Autodesk Inventor part; units mm, degrees
ref_plane "YZ Plane" through (0, 0, 0) normal (1, 0, 0) x (0, 1, 0)
ref_plane "XZ Plane" through (0, 0, 0) normal (0, 1, 0) x (-1, 0, 0)
ref_plane "XY Plane" through (0, 0, 0) normal (0, 0, 1) x (1, 0, 0)
sketch "Sketch1" plane through (0, 0, 0) normal (0, 0, 1) x (1, 0, 0)
  circle A0 centre (0, 0) radius 3.5
  dimension "d0" = 7
extrude "Extrusion1" add sketch "Sketch1" along normal blind 15
fillet "Fillet1" radius 2 1 edges at (-3.5, 0, 15)
hole "Hole1" at (0, 0, 0) direction (0, 0, 1) diameter 3.25 end through all
properties part number "Landing Gear"
Model file for the job. Use its own axes, mm. Give positions to 0.01 mm unless a question says otherwise; leave off trailing zeros. Order: outer loops, then holes, each group sorted by start corner. A loop starts at its lowest first (then second) coordinate and runs counter-clockwise, first axis right, second up. Notation, with made-up numbers: M -5.5,3.5 L 46.5,3.5 A23 ccw 46.5,23.5 Z; hole C -30,-39 d11. An arc over 180 degrees is marked long. Put each result on its own line as item: value. Start each with the question number.
(1) Pin check, flat tips, straight feed: pin 1 Ø1.5 at (x, z) = (1, 6) entering from +Y; pin 2 Ø1 at (x, z) = (-1.5, 8) entering from +Y; pin 3 Ø1 at (x, z) = (-2, 13) entering from +Y. Stop position of each tip, or through.
(2) Pull direction X, two halves, no side cores. Call faces 1 (the face through (0.99, -1.29, 7.6)), 2 (the face through (1, -2, 0)), 3 (the face through (3.233, 1.341, 6.409)): released by +X, released by -X, zero draft, split by the parting line, or undercut.
(3) Band-saw the part on A-A on z = 4. Give the cut face in (x, y) (3 decimals), then the cut area to 3 significant figures.
(4) Drill centre lines: L1, parallel to Y at x = 0, z = 8.75 (3 decimals); L2, parallel to Y at x = -0.5, z = 9.5; L3, parallel to X at y = 1, z = 2.5. Where is each one in solid material? Low to high. Write a range as [from, to].
Results below:
1. pin 1: stops at y = 3.49
1. pin 2: stops at y = 3.35
1. pin 3: stops at y = 3.16
2. face 1: undercut
2. face 2: zero draft
2. face 3: split by the parting line
3. outline: C 0,0 d7; hole C 0,0 d3.25
3. area: 30.2 mm2
4. L1: y = [-3.5, -1.625], [1.625, 3.5]
4. L2: y = [-3.46, -1.55], [1.55, 3.46]
4. L3: x = [-3.35, -1.28], [1.28, 3.35]
